CAD build for the part. Positions are in the model's coordinates, mm. Coordinates: 2 decimals unless noted, no trailing zeros. Write each loop counter-clockwise with the first axis right and the second up, starting at its lowest first coordinate (ties: lowest second). Pieces come first, ordered by that corner, then holes. Notation, with made-up numbers: (35.5, 4.25) - (75.5, 4.25) arc R16 cw to (75.5, 11.25) - close; hole circle Ø10 at (5.5, -3). An arc over 180 degrees is marked (long way). Answer in a Markdown table with one row per item. Add a question column.
Q1. Band-saw the part on B-B (x = 389.5). List the corners of the cut face in (y, z), and give its area (3 significant figures).
Q2. Pin check, flat tips, straight feed: pin 1 (1 mm diameter, centred on y = 100, z = 2, fed in from -X); pin 2 (1 mm diameter, centred on x = -97.5, z = 3.5, fed in from -Y). Stop position of each tip, or through.
Q3. Band-saw the part on C-C (y = -514). List the corners of the cut face in (x, z).
Q4. Drill centre lines: line 1 along Y through (x, z) = (8.5, 2.55); line 2 along X through (y, z) = (0, 2.4); line 3 along X through (y, z) = (-19, 2.15). Where is each one in solid material? Low to high. Write a range as from..to.
Q5. Band-saw the part on A-A (z = 2). List the corners of the cut face in (x, y).
```python
from build123d import *

# Parameters (mm, degrees)
F1_DEPTH = 4
F3_DEPTH = 25


with BuildPart() as f1:
    # F0 (on Top) → F1 (new body)
    with BuildSketch(Plane.XY):
        with BuildLine():
            Line((543.323108, 495), (-543.323108, 495))
            ThreePointArc((-543.323108, 495), (0, -735), (543.323108, 495))
        make_face()
    extrude(amount=F1_DEPTH)

    # F2 (on face) → F3 (cut)
    with BuildSketch(Plane.XY.offset(4)):
        with BuildLine():
            Line((21, -616.5), (-21, -616.5))
            ThreePointArc((-21, -616.5), (-25.5, -621), (-21, -625.5))
            Line((-21, -625.5), (21, -625.5))
            ThreePointArc((21, -625.5), (25.5, -621), (21, -616.5))
        make_face()
        with BuildLine():
            Line((21, -641.5), (-21, -641.5))
            ThreePointArc((-21, -641.5), (-25.5, -646), (-21, -650.5))
            Line((-21, -650.5), (21, -650.5))
            ThreePointArc((21, -650.5), (25.5, -646), (21, -641.5))
        make_face()
    extrude(amount=-F3_DEPTH, mode=Mode.SUBTRACT)


solid = f1.part
```
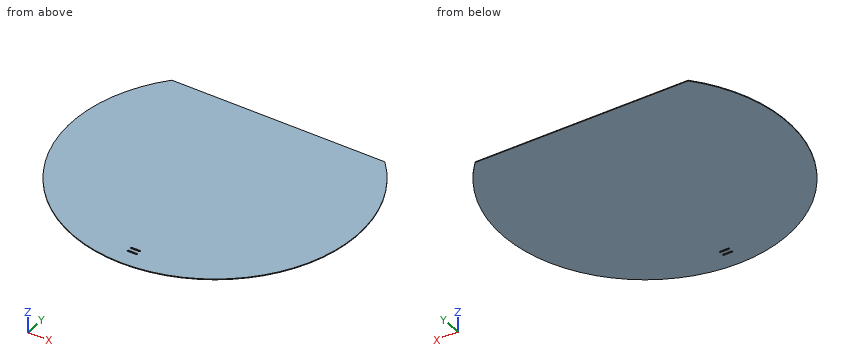
Checked values:
| question | item | result |
|---|---|---|
| 1 | outline | (-623.31, 0) - (495, 0) - (495, 4) - (-623.31, 4) - close |
| 1 | area | 4,470 mm² |
| 2 | pin 1 | stops at x = -728.23 |
| 2 | pin 2 | stops at y = -728.57 |
| 3 | outline | (-525.38, 0) - (525.38, 0) - (525.38, 4) - (-525.38, 4) - close |
| 4 | line 1 | y = -734.95..-650.5, -641.5..-625.5, -616.5..495 |
| 4 | line 2 | x = -735..735 |
| 4 | line 3 | x = -734.75..734.75 |
| 5 | outline | (-543.32, 495) arc R735 ccw (long way) to (543.32, 495) - close; hole (-21, -650.5) - (21, -650.5) arc R4.5 ccw to (21, -641.5) - (-21, -641.5) arc R4.5 ccw to start; hole (-21, -625.5) - (21, -625.5) arc R4.5 ccw to (21, -616.5) - (-21, -616.5) arc R4.5 ccw to start |
